```python
from build123d import *

# Parameters (mm, degrees)
SKETCH1_W           = 5.08
SKETCH1_H           = 13.97
SKETCH1_W_2         = 53.34
SKETCH1_H_2         = 43.18
SKETCH1_W_3         = 15.946260678
SKETCH1_H_3         = 5.08
BOSS_EXTRUDE1_DEPTH = 5.588


with BuildPart() as part:
    # Sketch1 → Boss-Extrude1 (new body)
    with BuildSketch(Plane.XY):
        with Locations((-29.21, 14.605)):
            Rectangle(SKETCH1_W, SKETCH1_H)
        Rectangle(SKETCH1_W_2, SKETCH1_H_2)
        with Locations((-0.487430597, 24.13)):
            Rectangle(SKETCH1_W_3, SKETCH1_H_3)
        with Locations((29.21, 14.605)):
            Rectangle(SKETCH1_W, SKETCH1_H)
        with Locations((-0.487430597, -24.13)):
            Rectangle(SKETCH1_W_3, SKETCH1_H_3)
        with Locations((-29.21, -14.605)):
            Rectangle(SKETCH1_W, SKETCH1_H)
        with Locations((29.21, -14.605)):
            Rectangle(SKETCH1_W, SKETCH1_H)
    extrude(amount=BOSS_EXTRUDE1_DEPTH)


solid = part.part
```
Source: CAD feature listing. Evaluate the final solid. Frame: model axes, mm. A direction names the side the tool comes from. Coordinates: 2 decimals unless noted, no trailing zeros. Loops run counter-clockwise (first coordinate to the right, second up) from the corner with the lowest first, then second, coordinate; pieces in that order, holes last. Notation, with made-up numbers: (-30.75, 86) -> (-7.75, 86) arc R22 cw to (-7.75, 98) -> close; hole circle Ø7 at (38, 85.25). An arc over 180 degrees is marked (long way). One line per item, written item: value. Start each with the question number.
Q1. Line query: line 1 along Y through (x, z) = (29.5, 1.3); line 2 along Y through (x, z) = (14, 0.55); line 3 along X through (y, z) = (-23, 1.75). Output: solid intervals per line, ascending.
Q2. Section query B-B, the plane x = 23. Return the cut outline in (y, z).
Q3. Mould query, pull axis Y, two halves, no side actions, for faces 1 (the face through (31.75, 15, 3)), 2 (the face through (-1, -26.67, 3)), 3 (the face through (26.67, 0, 3)). Classes: pulls with the +Y half, pulls with the -Y half, needs draft (parallel to the pull), parting line crosses it, or undercut.
Q4. Set-up query: faces 4 (the face through (-20, 21.59, 3)), 5 (the face through (29, -7.62, 3)), 6 (the face through (19, -21.59, 3)), 7 (the face through (-26.67, 0, 3)). Return all of +Z, -Z, +X, -X, +Y, -Y with unobstructed straight access to the full face (end or side cutting, diameter ignored); none if empty.
Q5. Contact query for flat-ended pins moving along their axis: P1, Ø1.5, axis at y = -24.5, z = 3.5, coming from the -X side; P2, Ø3, axis at x = -19.5, z = 2.5, coming from the -Y side; P3, Ø1.5, axis at y = 24.5, z = 2, coming from the +X side. Output: stop coordinate, or through.
Q6. Section query C-C, the plane y = 2.5. Return the cut outline in (x, z).
Q7. Section query A-A, the plane z = 3.75. Return the cut outline in (x, y), and give its area (3 significant figures).
Results:
1. line 1: -21.59 to -7.62, 7.62 to 21.59
1. line 2: -21.59 to 21.59
1. line 3: -8.46 to 7.49
2. outline: (-21.59, 0) -> (21.59, 0) -> (21.59, 5.59) -> (-21.59, 5.59) -> close
3. face 1: needs draft
3. face 2: pulls with the -Y half
3. face 3: undercut
4. face 4: +Z, -Z, -X, +Y
4. face 5: +Z, -Z, +X
4. face 6: +Z, -Z, +X, -Y
4. face 7: +Z, -Z, -X
5. P1: x = -8.46
5. P2: y = -21.59
5. P3: x = 7.49
6. outline: (-26.67, 0) -> (26.67, 0) -> (26.67, 5.59) -> (-26.67, 5.59) -> close
7. outline: (-31.75, -21.59) -> (-8.46, -21.59) -> (-8.46, -26.67) -> (7.49, -26.67) -> (7.49, -21.59) -> (31.75, -21.59) -> (31.75, -7.62) -> (26.67, -7.62) -> (26.67, 7.62) -> (31.75, 7.62) -> (31.75, 21.59) -> (7.49, 21.59) -> (7.49, 26.67) -> (-8.46, 26.67) -> (-8.46, 21.59) -> (-31.75, 21.59) -> (-31.75, 7.62) -> (-26.67, 7.62) -> (-26.67, -7.62) -> (-31.75, -7.62) -> close
7. area: 2,750 mm^2
